Here's how the part is built. I have some questions about the finished solid (model axes, mm). A direction names the side the tool comes from. Give positions to 0.01 mm unless a question says otherwise; leave off trailing zeros. Order: outer loops, then holes, each group sorted by start corner. A loop starts at its lowest first (then second) coordinate and runs counter-clockwise, first axis right, second up.
from build123d import *

# Parameters (mm, degrees)
SKETCH1_W           = 50.8
SKETCH1_H           = 31.75
BOSS_EXTRUDE1_DEPTH = 25.4
FILLET1_R           = 5.08


with BuildPart() as part:
    # Sketch1 → Boss-Extrude1 (new body)
    with BuildSketch(Plane.XY):
        Polygon((-101.6, -3.175), (-31.75, -3.175), (-102.245124878, -28.833127117), (-99.933913891, -35.183127117), (-31.75, -10.366212005), (-31.75, -22.225), (-8.889749428, -22.225), (-75.27486339, -85.781410988), (-75.27486339, -95.016274378), (-2.54, -22.281410988), (-2.54, -98.481410988), (2.54, -98.481410988), (2.54, -22.281410988), (75.27486339, -95.016274378), (75.27486339, -85.781410988), (8.889749428, -22.225), (31.75, -22.225), (31.75, -10.366212005), (99.933913891, -35.183127117), (102.245124878, -28.833127117), (31.75, -3.175), (101.6, -3.175), (101.6, 3.175), (31.75, 3.175), (102.245124878, 28.833127117), (99.933913891, 35.183127117), (31.75, 10.366212005), (31.75, 22.225), (8.948671098, 22.225), (75.27486339, 85.725), (75.27486339, 94.95986339), (2.54, 22.225), (2.54, 98.425), (-2.54, 98.425), (-2.54, 22.225), (-75.27486339, 94.95986339), (-75.27486339, 85.725), (-8.948671098, 22.225), (-31.75, 22.225), (-31.75, 10.366212005), (-99.933913891, 35.183127117), (-102.245124878, 28.833127117), (-31.75, 3.175), (-101.6, 3.175), align=None)
        Rectangle(SKETCH1_W, SKETCH1_H, mode=Mode.SUBTRACT)
    extrude(amount=BOSS_EXTRUDE1_DEPTH)

    # Fillet1
    fillet1_edges = [part.edges().sort_by_distance(p)[0] for p in [
        (31.75, -22.225, 12.7),
        (-31.75, -22.225, 12.7),
        (-31.75, 22.225, 12.7),
        (31.75, 22.225, 12.7),
    ]]
    fillet(fillet1_edges, radius=FILLET1_R)


solid = part.part
Q1. For faces 1 (the face through (-41.62, -53.56, 12.52)), 2 (the face through (-39.42, -59.16, 12.52)), 3 (the face through (2.54, 60, 13)), 4 (the face through (66.504, 15.824, 12.522)), 5 (the face through (-75.275, -90, 13)), which set-ups out of +Z, -Z, +X, -X, +Y, -Y let a thin tool reach every point of the face, with its end or its side?
Filled sheet:
face 1: +Z, -Z
face 2: +Z, -Z, -Y
face 3: +Z, -Z, +Y
face 4: +Z, -Z, +X
face 5: +Z, -Z, -X, -Y
Q2. If we section it at D-D on x = -82.5: List the corners of the cut face in (y, z) for me (3 decimals), plus the area to 3 significant figures.
Filled sheet:
outline: (-28.838, 0) - (-21.646, 0) - (-21.646, 25.4) - (-28.838, 25.4) - close; (-3.175, 0) - (3.175, 0) - (3.175, 25.4) - (-3.175, 25.4) - close; (21.646, 0) - (28.838, 0) - (28.838, 25.4) - (21.646, 25.4) - close
area: 527 mm2
Q3. I'm going to push flat-ended pins straight in: P1, Ø12, axis at x = 19.5, y = -53.5, coming from the +Z side; P2, Ø3, axis at y = -77, z = 11, coming from the +X side; P3, Ø14, axis at x = -17.5, z = 15.5, coming from the -Y side; P4, Ø7.5, axis at y = -90, z = 9, coming from the +X side. Where does each tip first touch, or does it pass through?
Filled sheet:
P1: passes through
P2: stops at x = 67.67
P3: stops at y = -44.24
P4: stops at x = 75.27
Q4. I need wall thicknesses on L1, parallel to X at y = 36.5, z = 3.25 (3 decimals); L2, parallel to Y at x = -18, z = 23.75 (3 decimals); L3, parallel to Y at x = -28, z = 13 (3 decimals). Which ranges of each line are inside material? Lowest first, please.
Filled sheet:
L1: x = -23.859 to -16.815, -2.54 to 2.54, 16.815 to 23.859
L2: y = -37.741 to -30.947, -22.225 to -15.875, 15.875 to 22.225, 30.891 to 37.685
L3: y = -47.741 to -40.521, -22.048 to 22.048, 40.465 to 47.685
Q5. If we section it at C-C on y = 31.5: List the corners of the cut face in (x, z) for me (3 decimals), plus the area to 3 significant figures.
Filled sheet:
outline: (-101.274, 0) - (-89.815, 0) - (-89.815, 25.4) - (-101.274, 25.4) - close; (-18.636, 0) - (-11.815, 0) - (-11.815, 25.4) - (-18.636, 25.4) - close; (-2.54, 0) - (2.54, 0) - (2.54, 25.4) - (-2.54, 25.4) - close; (11.815, 0) - (18.636, 0) - (18.636, 25.4) - (11.815, 25.4) - close; (89.815, 0) - (101.274, 0) - (101.274, 25.4) - (89.815, 25.4) - close
area: 1,060 mm2
Q6. If we section it at A-A on y = 6: List the corners of the cut face in (x, z) for me.
Filled sheet:
outline: (-39.51, 0) - (-25.4, 0) - (-25.4, 25.4) - (-39.51, 25.4) - close; (25.4, 0) - (39.51, 0) - (39.51, 25.4) - (25.4, 25.4) - close
Q7. If we section it at B-B on x = -60: List the corners of the cut face in (y, z) for me (3 decimals).
Filled sheet:
outline: (-79.741, 0) - (-71.157, 0) - (-71.157, 25.4) - (-79.741, 25.4) - close; (-20.648, 0) - (-13.457, 0) - (-13.457, 25.4) - (-20.648, 25.4) - close; (-3.175, 0) - (3.175, 0) - (3.175, 25.4) - (-3.175, 25.4) - close; (13.457, 0) - (20.648, 0) - (20.648, 25.4) - (13.457, 25.4) - close; (71.101, 0) - (79.685, 0) - (79.685, 25.4) - (71.101, 25.4) - close
